```python
from build123d import *

# Parameters (mm, degrees)
SKETCH_2_OUTSIDE_W  = 29.51
SKETCH_2_OUTSIDE_H  = 29.51
CUT_EXTRUDE_1_DEPTH = 44.997697667
CHAMFER_1_SIZE      = 1


with BuildPart() as part:
    # Эскиз1 → Повернуть1 (revolve)
    with BuildSketch(Plane.XY, mode=Mode.PRIVATE) as revolve_1_sk:
        Polygon((-6.58, 0), (-6.58, 8.85), (0, 8.85), (0, 7.448974596), (0.6, 7.288205081), (0.6, 5), (35.6, 5), (35.6, 0), align=None)
    revolve(revolve_1_sk.sketch.rotate(Axis((-1000, 0, 0), (1, 0, 0)), 90), axis=Axis((-1000, 0, 0), (1, 0, 0)))

    # Эскиз2 outside → Вырез-Вытянуть1 (cut, through all)
    with BuildSketch(Plane.ZY.offset(6.58)):
        Rectangle(SKETCH_2_OUTSIDE_W, SKETCH_2_OUTSIDE_H)
        Polygon((0, -8.85), (7.664324823, -4.425), (7.664324823, 4.425), (0, 8.85), (-7.664324823, 4.425), (-7.664324823, -4.425), align=None, mode=Mode.SUBTRACT)
    extrude(amount=-CUT_EXTRUDE_1_DEPTH, mode=Mode.SUBTRACT)

    # Эскиз4 → Вырез-Повернуть1 (revolve, cut)
    with BuildSketch(Plane.XY):
        Polygon((-6.58, 8.075), (-6.297923068, 8.85), (-6.58, 8.85), align=None)
    revolve(axis=Axis((-1000, 0, 0), (1, 0, 0)), mode=Mode.SUBTRACT)

    # Фаска1
    chamfer_1_edges = [part.edges().sort_by_distance(p)[0] for p in [
        (35.6, 0, -5),
    ]]
    chamfer(chamfer_1_edges, length=CHAMFER_1_SIZE)


solid = part.part
```
Model file for the job. Use its own axes, mm. A direction names the side the tool comes from. Coordinates: 2 decimals unless noted, no trailing zeros. Write each loop counter-clockwise with the first axis right and the second up, starting at its lowest first coordinate (ties: lowest second). Pieces come first, ordered by that corner, then holes. Notation, with made-up numbers: (-12, 22.25) - (-3, 22.25) arc R26 cw to (-3, 59.25) - close; hole circle Ø6 at (61.25, -11.5). An arc over 180 degrees is marked (long way). Use a Markdown table: item, result. Add a question column.
Item 1: 3-axis set-ups, long thin cutter, end or side, ignore diameter. For faces 1 (the face through (-6.5, 8.3, 0)), 2 (the face through (18, 0, -5)): which of +Z, -Z, +X, -X, +Y, -Y reach the whole face in a straight line?
Item 2: Band-saw the part on B-B, the plane x = 26.5. Write the cut outline in (y, z), and give its area (3 significant figures).
Item 3: Drill centre lines: line 1 along Z through (x, y) = (16.5, -0.25); line 2 along X through (y, z) = (-6.5, -1); line 3 along X through (y, z) = (-5.25, 5.75). Where is each one in solid material? Low to high.
Item 4: Drop flat-ended pins along their axis: pin 1 (8 mm diameter, centred on y = 5.5, z = 2.5, fed in from +X); pin 2 (3 mm diameter, centred on x = 3.5, z = 3, fed in from -Y); pin 3 (3 mm diameter, centred on x = 26.5, y = 4, fed in from -Z). Give the stop position or say it passes through.
Item 5: Band-saw the part on A-A, the plane y = 0. Write the cut outline in (x, z), and give its area (3 significant figures).
Item 6: Two-plate mould, pull along X, no slides. Class faces 3 (the face through (35.6, 0, 0)), 4 (the face through (-3.3, 6.6, 3.9)), 5 (the face through (-6.5, 4.17, 7.17)): pulls with the +X half, pulls with the -X half, needs draft (parallel to the pull), parting line crosses it, or undercut.
A:
| question | item | result |
|---|---|---|
| 1 | face 1 | -X, +Y |
| 1 | face 2 | +X |
| 2 | outline | circle Ø10 at (0, 0) |
| 2 | area | 78.5 mm² |
| 3 | line 1 | z = -4.99 to 4.99 |
| 3 | line 2 | x = -6.58 to 0.6 |
| 3 | line 3 | x = -6.58 to 0 |
| 4 | pin 1 | stops at x = 35.6 |
| 4 | pin 2 | stops at y = -4.77 |
| 4 | pin 3 | stops at z = -4.33 |
| 5 | outline | (-6.58, -7.66) - (0, -7.66) - (0, -7.45) - (0.6, -7.29) - (0.6, -5) - (34.6, -5) - (35.6, -4) - (35.6, 4) - (34.6, 5) - (0.6, 5) - (0.6, 7.29) - (0, 7.45) - (0, 7.66) - (-6.58, 7.66) - close |
| 5 | area | 459 mm² |
| 6 | face 3 | pulls with the +X half |
| 6 | face 4 | needs draft |
| 6 | face 5 | pulls with the -X half |
